Check sheet for the modelled part. Datum: model origin and axes. Units: mm. A direction names the side the tool comes from. Coordinates: 2 decimals unless noted, no trailing zeros. Write each loop counter-clockwise with the first axis right and the second up, starting at its lowest first coordinate (ties: lowest second). Pieces come first, ordered by that corner, then holes. Notation, with made-up numbers: (5, 51) - (57, 51) arc R17 cw to (57, 79) - close; hole circle Ø4 at (-29, 25). An arc over 180 degrees is marked (long way). Write each question's results on one line, items separated by ' | '.
from build123d import *

# Parameters (mm, degrees)
SKETCH1_W           = 45
SKETCH1_H           = 150
BOSS_EXTRUDE1_DEPTH = 4
SKETCH2_R           = 22.5
BOSS_EXTRUDE2_DEPTH = 4
SKETCH3_R           = 2.25
CUT_EXTRUDE1_DEPTH  = 5
CIRPATTERN1_COUNT   = 6
SKETCH4_R           = 1.75
CUT_EXTRUDE2_DEPTH  = 4
CIRPATTERN2_COUNT   = 3
CUT_EXTRUDE3_DEPTH  = 4


with BuildPart() as part:
    # Sketch1 → Boss-Extrude1 (new body)
    with BuildSketch(Plane(origin=(0, 0, 0), x_dir=(1, 0, 0), z_dir=(0, 1, 0))):
        Rectangle(SKETCH1_W, SKETCH1_H)
    extrude(amount=BOSS_EXTRUDE1_DEPTH)

    # Sketch2 → Boss-Extrude2 (add)
    with BuildSketch(Plane(origin=(0, 0, 0), x_dir=(1, 0, 0), z_dir=(0, 1, 0))):
        with Locations((0, 75)):
            Circle(SKETCH2_R)
    extrude(amount=BOSS_EXTRUDE2_DEPTH)

    # Sketch3 → Cut-Extrude1 (cut, through all)
    with BuildSketch(Plane(origin=(0, 4, 0), x_dir=(1, 0, 0), z_dir=(0, 1, 0))):
        with Locations((0, 84.5)):
            Circle(SKETCH3_R)
    cut_extrude1 = extrude(amount=-CUT_EXTRUDE1_DEPTH, mode=Mode.SUBTRACT)

    # CirPattern1: Cut-Extrude1 ×6 about axis
    cirpattern1_axis = Axis((0, 0, -75), (0, 1, 0))
    for i in range(1, CIRPATTERN1_COUNT):
        add(cut_extrude1.rotate(cirpattern1_axis, i * 360 / CIRPATTERN1_COUNT), mode=Mode.SUBTRACT)

    # Sketch4 → Cut-Extrude2 (cut)
    with BuildSketch(Plane(origin=(0, 4, 0), x_dir=(1, 0, 0), z_dir=(0, 1, 0))):
        with Locations((0, 72)):
            Circle(SKETCH4_R)
    cut_extrude2 = extrude(amount=-CUT_EXTRUDE2_DEPTH, mode=Mode.SUBTRACT)

    # CirPattern2: Cut-Extrude2 ×3 about axis
    cirpattern2_axis = Axis((0, 0, -75), (0, 1, 0))
    for i in range(1, CIRPATTERN2_COUNT):
        add(cut_extrude2.rotate(cirpattern2_axis, i * 360 / CIRPATTERN2_COUNT), mode=Mode.SUBTRACT)

    # Sketch5 → Cut-Extrude3 (cut)
    with BuildSketch(Plane(origin=(0, 4, 0), x_dir=(1, 0, 0), z_dir=(0, 1, 0))):
        with BuildLine():
            Line((-6.75, -10), (-6.75, -60))
            ThreePointArc((-6.75, -60), (-10, -63.25), (-13.25, -60))
            Line((-13.25, -60), (-13.25, -10))
            ThreePointArc((-13.25, -10), (-10, -6.75), (-6.75, -10))
        make_face()
    cut_extrude3 = extrude(amount=-CUT_EXTRUDE3_DEPTH, mode=Mode.SUBTRACT)

    # Mirror1: Cut-Extrude3 across plane
    add(cut_extrude3.mirror(Plane(origin=(0, 0, 0), x_dir=(0, 0, 1), z_dir=(1, 0, 0))), mode=Mode.SUBTRACT)


solid = part.part
1. Draft check along X on faces 3 (the cylindrical face through (9.265, 2.028, -68.254)), 4 (the cylindrical face through (0.495, 1.972, -97.495)), 5 (the flat face through (0, 2, 75)). Enter one of: pulls with the +X half, pulls with the -X half, needs draft (parallel to the pull), parting line crosses it, or undercut.
Values follow:
face 3: undercut | face 4: parting line crosses it | face 5: needs draft
2. Access from +Z, -Z, +X, -X, +Y, -Y to the whole of each face (thin tool, end or side, straight path). Record for faces 1 (the flat face through (-6.75, 2, 35)), 2 (the flat face through (-22.5, 2, 1)).
Values follow:
face 1: +Y, -Y | face 2: +Z, -Z, -X, +Y, -Y
3. Sectioned sample at A-A (z = 18). Record the cut outline in (x, y), then the cut area to 3 significant figures.
Values follow:
outline: (-22.5, 0) - (-13.25, 0) - (-13.25, 4) - (-22.5, 4) - close; (-6.75, 0) - (6.75, 0) - (6.75, 4) - (-6.75, 4) - close; (13.25, 0) - (22.5, 0) - (22.5, 4) - (13.25, 4) - close | area: 128 mm^2
4. Sectioned sample at B-B (y = 2). Give the number of separate pieces and of enclosed holes in the cut face, then the cut area to 3 significant figures.
Values follow:
separate pieces: 1 | enclosed holes: 11 | area: 6,700 mm^2
5. Sectioned sample at C-C (x = -15). Record the cut outline in (y, z).
Values follow:
outline: (0, -91.77) - (4, -91.77) - (4, 75) - (0, 75) - close
6. Material ranges on L1, parallel to Z at x = 0, y = 0.4; L2, parallel to X at y = 2.45, z = -79.75; L3, parallel to Z at x = -1, y = 1.1, recorded low to high. Write a range as [from, to].
Values follow:
L1: z = [-97.5, -86.75], [-82.25, -73.75], [-70.25, -67.75], [-63.25, 75] | L2: x = [-21.99, -10.48], [-5.98, 5.98], [10.48, 21.99] | L3: z = [-97.48, -86.52], [-82.48, -77.21], [-75.79, -73.44], [-70.56, -67.52], [-63.48, 75]
